Autodesk Inventor part; units mm, degrees
ref_plane "YZ Plane" through (0, 0, 0) normal (1, 0, 0) x (0, 1, 0)
ref_plane "XZ Plane" through (0, 0, 0) normal (0, 1, 0) x (-1, 0, 0)
ref_plane "XY Plane" through (0, 0, 0) normal (0, 0, 1) x (1, 0, 0)
sketch "Sketch1" plane through (0, 0, 0) normal (0, 0, 1) x (1, 0, 0)
  circle A0 centre (0, 0) radius 2.1844
  circle A1 centre (76.2, 0) radius 2.1844
  circle A2 centre (25.4, 0) radius 2.1844
  circle A3 centre (50.8, 0) radius 2.1844
  line L0 (0, -6.35) -> (76.2, -6.35)
  arc A4 (76.2, -6.35) -> (76.2, 6.35) centre (76.2, 0) ccw
  line L1 (76.2, 6.35) -> (0, 6.35)
  arc A5 (0, 6.35) -> (0, -6.35) centre (0, 0) ccw
  dimension "d0" = 4.3688
  dimension "d6" = 4.3688
  dimension "d12" = 4.3688
  dimension "d13" = 25.4
  dimension "d14" = 76.2
  dimension "d15" = 4.3688
  dimension "d16" = 25.4
  dimension "d17" = 76.2
  dimension "d20" = 76.2
extrude "Extrusion2" add sketch "Sketch1" along normal blind 1.5875
properties part number "2ndpreroller" material "Polycarbonate, Clear"
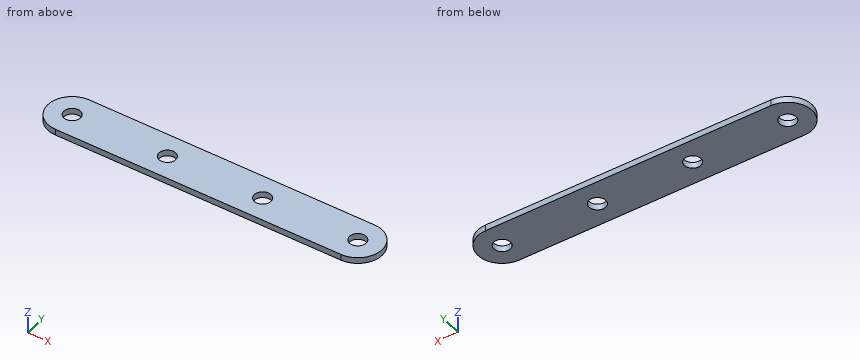
Could you check a few things on this model? Use its own coordinates, in mm. Coordinates: 2 decimals unless noted, no trailing zeros. Write each loop counter-clockwise with the first axis right and the second up, starting at its lowest first coordinate (ties: lowest second). Pieces come first, ordered by that corner, then holes. Notation, with made-up numbers: (-6.75, -8.5) - (14.25, -8.5) arc R33 cw to (14.25, 19.5) - close; hole circle Ø2 at (68, 57). An arc over 180 degrees is marked (long way). Write item = value, one per line.
1) Suppose I cut it at D-D on y = -4.25. Please give me the cut outline in (x, z), plus the area to 3 significant figures.
Result set:
outline = (-4.72, 0) - (80.92, 0) - (80.92, 1.59) - (-4.72, 1.59) - close
area = 136 mm2
2) Suppose I cut it at C-C on z = 0.4. Please give me the cut outline in (x, y).
Result set:
outline = (0, -6.35) - (76.2, -6.35) arc R6.35 ccw to (76.2, 6.35) - (0, 6.35) arc R6.35 ccw to start; hole circle Ø4.37 at (0, 0); hole circle Ø4.37 at (25.4, 0); hole circle Ø4.37 at (50.8, 0); hole circle Ø4.37 at (76.2, 0)
3) Suppose I cut it at A-A on x = 25.4. Please give me the cut outline in (y, z).
Result set:
outline = (-6.35, 0) - (-2.18, 0) - (-2.18, 1.59) - (-6.35, 1.59) - close; (2.18, 0) - (6.35, 0) - (6.35, 1.59) - (2.18, 1.59) - close
4) Please list where these lines run through material, in increasing order: line 1 (Y direction, x = 76.2, z = 1.25); line 2 (X direction, y = -1, z = 0.7). Write a range as [from, to].
Result set:
line_1 = [-6.35, -2.18], [2.18, 6.35]
line_2 = [-6.27, -1.94], [1.94, 23.46], [27.34, 48.86], [52.74, 74.26], [78.14, 82.47]
5) Suppose I cut it at B-B on y = 0. Please give me the cut outline in (x, z), plus the area to 3 significant figures.
Result set:
outline = (-6.35, 0) - (-2.18, 0) - (-2.18, 1.59) - (-6.35, 1.59) - close; (2.18, 0) - (23.22, 0) - (23.22, 1.59) - (2.18, 1.59) - close; (27.58, 0) - (48.62, 0) - (48.62, 1.59) - (27.58, 1.59) - close; (52.98, 0) - (74.02, 0) - (74.02, 1.59) - (52.98, 1.59) - close; (78.38, 0) - (82.55, 0) - (82.55, 1.59) - (78.38, 1.59) - close
area = 113 mm2
